Geometry check sheet. Reference: the model listing, model coordinates, mm. Face numbers are marked on the shaded views. A direction names the side the tool comes from. Round coordinates to 2 decimals unless told otherwise and drop trailing zeros. Order: outer loops, then holes, each group sorted by start corner. A loop starts at its lowest first (then second) coordinate and runs counter-clockwise, first axis right, second up. Notation, with made-up numbers: (-1.75, 50.5) - (16.25, 50.5) arc R12 ccw to (16.25, 59.5) - close; hole circle Ø9 at (39, 66.25). An arc over 180 degrees is marked (long way). Use a Markdown table: item, result. Add a question column.
(1) Mould release check, pull along Z, two halves, no side actions. Record for the marked faces 3, 4 and 5: released by +Z, released by -Z, zero draft, split by the parting line, or undercut.
(2) Section check A-A on z = 0. Record the boundary of the cut face in (x, y) (3 decimals).
(3) Section check C-C on y = -6.5. Record the boundary of the cut face in (x, z) (3 decimals).
(4) Thickness scan on line 1 along X through (y, z) = (2.6, 0); line 2 along Y through (x, z) = (-1.9, -0.6); line 3 along X through (y, z) = (1.25, -1.7). Record the ranges inside material, lowest first. Write a range as [from, to].
(5) Section check B-B on x = 0. Record the boundary of the cut face in (y, z) (3 decimals), then the cut area to 3 significant figures.
(6) Gauge pin test, flat ends, axial feed: P1, Ø1, axis at x = -1.5, z = 0, coming from the -Y side; P2, Ø1, axis at x = 1.5, y = -1, coming from the +Z side (3 decimals); P3, Ø3, axis at y = -3, z = -1, coming from the -X side (3 decimals); P4, Ø2, axis at x = -2, y = -10, coming from the +Z side. Record the tip position at first contact, or that the pin passes through.
(7) Access from +Z, -Z, +X, -X, +Y, -Y to the whole of each face (thin tool, end or side, straight path). Record for the marked faces 1 and 2.
```python
from build123d import *

# Parameters (mm, degrees)
BOSS_EXTRUDE1_DEPTH = 0.24
SKETCH3_R           = 2.35
BOSS_EXTRUDE2_DEPTH = 2.44
SKETCH4_R           = 1
CUT_EXTRUDE1_DEPTH  = 0.2794
SKETCH6_R           = 0.225
BOSS_EXTRUDE3_DEPTH = 13.2
FILLET1_R           = 0.25


with BuildPart() as part:
    # Sketch1 → Boss-Extrude1 (new body)
    with BuildSketch(Plane(origin=(0, 0, 0), x_dir=(1, 0, 0), z_dir=(0, 1, 0))):
        with BuildLine():
            Line((-2.234301709, -1.51588122), (-2.952722199, -2.234301709))
            Line((-2.952722199, -2.234301709), (-2.234301709, -2.952722199))
            Line((-2.234301709, -2.952722199), (-1.51588122, -2.234301709))
            ThreePointArc((-1.51588122, -2.234301709), (1.909188309, 1.909188309), (-2.234301709, -1.51588122))
        make_face()
    extrude(amount=BOSS_EXTRUDE1_DEPTH)

    # Sketch3 → Boss-Extrude2 (add)
    with BuildSketch(Plane(origin=(0, 0.24, 0), x_dir=(1, 0, 0), z_dir=(0, 1, 0))):
        with Locations(Location((0, 0, 0), (0, 0, 270))):  # turned: the seam where the file's is
            Circle(SKETCH3_R)
    extrude(amount=BOSS_EXTRUDE2_DEPTH)

    # Sketch4 → Cut-Extrude1 (cut)
    with BuildSketch(Plane(origin=(0, 2.68, 0), x_dir=(1, 0, 0), z_dir=(0, 1, 0))):
        with Locations(Location((0, 0, 0), (0, 0, 270))):  # turned: the seam where the file's is
            Circle(SKETCH4_R)
    extrude(amount=-CUT_EXTRUDE1_DEPTH, mode=Mode.SUBTRACT)

    # Sketch6 → Boss-Extrude3 (add)
    with BuildSketch(Plane.XZ):
        with Locations(Location((0, 1.27, 0), (0, 0, 90))):  # turned: the seam where the file's is
            Circle(SKETCH6_R)
        with Locations(Location((0, -1.27, 0), (0, 0, 90))):  # turned: the seam where the file's is
            Circle(SKETCH6_R)
        with Locations(Location((1.27, 0, 0), (0, 0, 90))):  # turned: the seam where the file's is
            Circle(SKETCH6_R)
    extrude(amount=BOSS_EXTRUDE3_DEPTH)

    # Fillet1
    fillet1_edges = [part.edges().sort_by_distance(p)[0] for p in [
        (0, 0.24, -2.35),
        (0, 2.68, -2.35),
    ]]
    fillet(fillet1_edges, radius=FILLET1_R)


solid = part.part
```
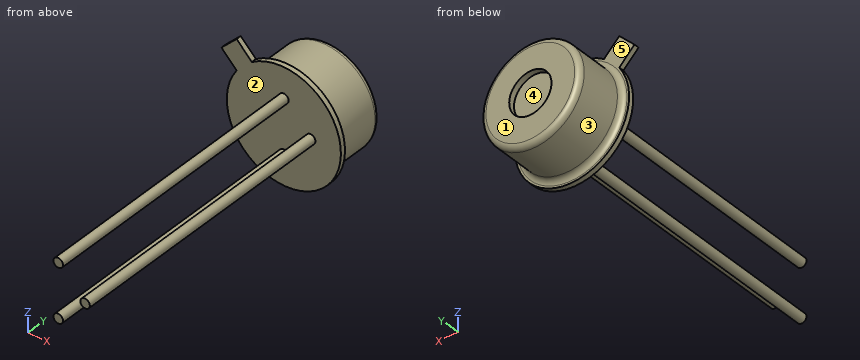
Check sheet entries:
| question | item | result |
|---|---|---|
| 1 | face 3 | split by the parting line |
| 1 | face 4 | undercut |
| 1 | face 5 | zero draft |
| 2 | outline | (-2.7, 0) - (1.045, 0) - (1.045, -13.2) - (1.495, -13.2) - (1.495, 0) - (2.7, 0) - (2.7, 0.24) - (2.6, 0.24) arc R0.25 cw to (2.35, 0.49) - (2.35, 2.43) arc R0.25 ccw to (2.1, 2.68) - (1, 2.68) - (1, 2.401) - (-1, 2.401) - (-1, 2.68) - (-2.1, 2.68) arc R0.25 ccw to (-2.35, 2.43) - (-2.35, 0.49) arc R0.25 cw to (-2.6, 0.24) - (-2.7, 0.24) - close |
| 3 | outline | circle Ø0.45 at (0, -1.27); circle Ø0.45 at (0, 1.27); circle Ø0.45 at (1.27, 0) |
| 4 | line 1 | x = [-2.28, -1], [1, 2.28] |
| 4 | line 2 | y = [0, 2.68] |
| 4 | line 3 | x = [-1.62, 1.62] |
| 5 | outline | (-13.2, -1.495) - (0, -1.495) - (0, -2.7) - (0.24, -2.7) - (0.24, -2.6) arc R0.25 cw to (0.49, -2.35) - (2.43, -2.35) arc R0.25 ccw to (2.68, -2.1) - (2.68, -1) - (2.401, -1) - (2.401, 1) - (2.68, 1) - (2.68, 2.1) arc R0.25 ccw to (2.43, 2.35) - (0.49, 2.35) arc R0.25 cw to (0.24, 2.6) - (0.24, 2.7) - (0, 2.7) - (0, 1.495) - (-13.2, 1.495) - (-13.2, 1.045) - (0, 1.045) - (0, -1.045) - (-13.2, -1.045) - close |
| 5 | area | 24.1 mm2 |
| 6 | P1 | stops at y = 0 |
| 6 | P2 | stops at z = 0.225 |
| 6 | P3 | stops at x = -0.225 |
| 6 | P4 | passes through |
| 7 | face 1 | +Z, -Z, +X, -X, +Y |
| 7 | face 2 | -Y |
